Read the model definition and answer for the solid it produces. Units are mm, in the model's axes. A direction names the side the tool comes from. Round coordinates to 2 decimals unless told otherwise and drop trailing zeros. Loops run counter-clockwise (first coordinate to the right, second up) from the corner with the lowest first, then second, coordinate; pieces in that order, holes last. Notation, with made-up numbers: M 84,57 L 92,57 A18 cw 92,92 Z; hole C 44.25,77.5 d4. An arc over 180 degrees is marked long. Write each question's results on one line, items separated by ' | '.
from build123d import *

# Parameters (mm, degrees)
SKETCH1_W                      = 665
SKETCH1_H                      = 650
BOSS_EXTRUDE1_DEPTH            = 30
F_8_0_199_DIAMETER_HOLE1_D     = 5.0546
F_8_0_199_DIAMETER_HOLE1_DEPTH = 9.65
SKETCH4_W                      = 615
SKETCH4_H                      = 600
CUT_EXTRUDE1_DEPTH             = 20


with BuildPart() as part:
    # Sketch1 → Boss-Extrude1 (new body)
    with BuildSketch(Plane(origin=(0, 0, 0), x_dir=(1, 0, 0), z_dir=(0, 1, 0))):
        with Locations((332.5, 325)):
            Rectangle(SKETCH1_W, SKETCH1_H)
    extrude(amount=-BOSS_EXTRUDE1_DEPTH)

    # #8 (0.199) Diameter Hole1
    with Locations(Plane(origin=(0, 0, 0), x_dir=(1, 0, 0), z_dir=(0, 1, 0))):
        with Locations((68.25, 13.5), (13.5, 301), (596.75, 13.5), (651.5, 301), (651.5, 349), (596.75, 636.5), (68.25, 636.5), (13.5, 349)):
            Hole(F_8_0_199_DIAMETER_HOLE1_D / 2, depth=F_8_0_199_DIAMETER_HOLE1_DEPTH)

    # Sketch4 → Cut-Extrude1 (cut)
    with BuildSketch(Plane(origin=(0, 0, 0), x_dir=(1, 0, 0), z_dir=(0, 1, 0))):
        with Locations((332.5, 325)):
            Rectangle(SKETCH4_W, SKETCH4_H)
    extrude(amount=-CUT_EXTRUDE1_DEPTH, mode=Mode.SUBTRACT)


solid = part.part
Item 1: The part is cut by section B-B (z = -422.5). Determine the outline of the cut face in (x, y), plus the area to 3 significant figures.
Outcome:
outline: M 0,-30 L 665,-30 L 665,0 L 640,0 L 640,-20 L 25,-20 L 25,0 L 0,0 Z | area: 7,650 mm2
Item 2: The part is cut by section A-A (x = 420). Determine the outline of the cut face in (y, z), plus the area to 3 significant figures.
Outcome:
outline: M -30,-650 L 0,-650 L 0,-625 L -20,-625 L -20,-25 L 0,-25 L 0,0 L -30,0 Z | area: 7,500 mm2
Item 3: Flat-ended cylindrical pins translate along their axes: pin 1 (4 mm diameter, centred on x = 67.5, z = -636.5, fed in from +Y); pin 2 (3 mm diameter, centred on x = 68.25, z = -13.5, fed in from +Y); pin 3 (3 mm diameter, centred on x = 558.5, z = -249, fed in from +Y). Find the tip coordinate at first contact, or state that the pin passes through.
Outcome:
pin 1: stops at y = 0 | pin 2: stops at y = -9.65 | pin 3: stops at y = -20
Item 4: For faces 1 (the face through (328, -20, -329)), 2 (the face through (328, -15, -650)), determine the directions among +Z, -Z, +X, -X, +Y, -Y from which every point of the face is accessible in a straight line to the end or side of a thin tool.
Outcome:
face 1: +Y | face 2: -Z, +X, -X, +Y, -Y
Item 5: Straight lines are drawn through the part: line 1 (Z direction, x = 68.25, y = -2.5); line 2 (X direction, y = -2.25, z = -349); line 3 (Z direction, x = 13.5, y = -3.5). For each, find the intervals that lie inside material, in ascending order.
Outcome:
line 1: z = -650 to -639.03, -633.97 to -625, -25 to -16.03, -10.97 to 0 | line 2: x = 0 to 10.97, 16.03 to 25, 640 to 648.97, 654.03 to 665 | line 3: z = -650 to -351.53, -346.47 to -303.53, -298.47 to 0
Item 6: The mould has two halves that part along X. Classify faces 3 (the face through (328, -10, -25)), 4 (the face through (665, -15, -320)), 5 (the face through (331, 0, -14)), 6 (the face through (25, -10, -321)): pulls with the +X half, pulls with the -X half, needs draft (parallel to the pull), parting line crosses it, or undercut.
Outcome:
face 3: undercut | face 4: pulls with the +X half | face 5: needs draft | face 6: undercut
